```python
from build123d import *

# Parameters (mm, degrees)
BOSS_EXTRUDE1_DEPTH      = 127
BOSS_EXTRUDE1_DEPTH_BACK = 127
SKETCH3_W                = 31.75
SKETCH3_H                = 31.75
SKETCH3_W_2              = 25.4
SKETCH3_H_2              = 25.4
F_10_CLEARANCE_HOLE1_D   = 4.9784
SKETCH7_R                = 14.2875
CUT_EXTRUDE1_DEPTH       = 7.62
CUT_EXTRUDE2_START       = -7.62
SKETCH8_R                = 14.2875
CUT_EXTRUDE2_DEPTH       = 7.62
CUT_EXTRUDE3_DEPTH       = 132.867653824
F_10_CLEARANCE_HOLE2_D   = 4.9784
SKETCH13_R               = 6.35
CUT_EXTRUDE4_DEPTH       = 132.867653824


with BuildPart() as part:
    # Sketch3 → Boss-Extrude1 (new, two sides: drawn at the far end of the back side and taken through both)
    with BuildSketch(Plane.XY.offset(-BOSS_EXTRUDE1_DEPTH_BACK)):
        Rectangle(SKETCH3_W, SKETCH3_H)
        Rectangle(SKETCH3_W_2, SKETCH3_H_2, mode=Mode.SUBTRACT)
    extrude(amount=BOSS_EXTRUDE1_DEPTH + BOSS_EXTRUDE1_DEPTH_BACK)

    # #10 Clearance Hole1 (through all)
    with Locations(Plane(origin=(0, 15.875, 0), x_dir=(1, 0, 0), z_dir=(0, 1, 0))):
        with Locations((-11.1125, -117.475), (11.1125, -117.475), (0, -98.247200001), (-7.111939052, -75.171256705)):
            Hole(F_10_CLEARANCE_HOLE1_D / 2)

    # Sketch7 → Cut-Extrude1 (cut)
    with BuildSketch(Plane(origin=(0, 15.875, 0), x_dir=(1, 0, 0), z_dir=(0, 1, 0))):
        with Locations(Location((0, 17.8816, 0), (0, 0, 270))):
            Circle(SKETCH7_R)
    extrude(amount=-CUT_EXTRUDE1_DEPTH, mode=Mode.SUBTRACT)

    # Sketch8 → Cut-Extrude2 (cut)
    with BuildSketch(Plane.XZ.offset(15.875).offset(CUT_EXTRUDE2_START)):
        with Locations(Location((0, -17.8816, 0), (0, 0, 90))):
            Circle(SKETCH8_R)
    extrude(amount=CUT_EXTRUDE2_DEPTH, mode=Mode.SUBTRACT)

    # Sketch9 → Cut-Extrude3 (cut, through all)
    with BuildSketch(Plane.XZ.offset(15.875)):
        with BuildLine():
            Line((-9.525, 27.51353779), (-9.525, 14.81353779))
            ThreePointArc((-9.525, 14.81353779), (-11.384871939, 10.323409729), (-15.875, 8.46353779))
            Line((-15.875, 8.46353779), (-15.875, 33.86353779))
            ThreePointArc((-15.875, 33.86353779), (-11.384871939, 32.00366585), (-9.525, 27.51353779))
        make_face()
    extrude(amount=-CUT_EXTRUDE3_DEPTH, mode=Mode.SUBTRACT)

    # #10 Clearance Hole2 (through all)
    with Locations(Plane(origin=(15.875, 0, 0), x_dir=(0, 0, -1), z_dir=(1, 0, 0))):
        with Locations((-82.55, 3.175), (114.3, 3.175), (40.132, 3.175)):
            Hole(F_10_CLEARANCE_HOLE2_D / 2)

    # Sketch13 → Cut-Extrude4 (cut, through all)
    with BuildSketch(Plane.XZ.offset(15.875)):
        with Locations((-20.955, 94.525686877)):
            Circle(SKETCH13_R)
    extrude(amount=-CUT_EXTRUDE4_DEPTH, mode=Mode.SUBTRACT)


solid = part.part
```
The listing builds one solid part. Answer for the finished solid, in the listing's coordinates (mm). A direction names the side the tool comes from. Coordinates: 2 decimals unless noted, no trailing zeros. Order: outer loops, then holes, each group sorted by start corner. A loop starts at its lowest first (then second) coordinate and runs counter-clockwise, first axis right, second up. Notation, with made-up numbers: M -2,50.25 L 34,50.25 A13 ccw 34,68.25 Z; hole C 45,82 d6. An arc over 180 degrees is marked long. Answer as a JSON object with one key per item and string values. Group by question number.
1. Determine the mould class of faces 5 (the flat face through (-15.875, 0, 112)), 6 (the cylindrical face through (-8.45, -14.31, 73.07)), 7 (the flat face through (-14, 0, -127)) for opening direction X: released by +X, released by -X, zero draft, split by the parting line, or undercut.
2. Section B-B on x = 0 is taken. Write down the section's boundary in (y, z) (3 decimals), then the cut area to 3 significant figures.
3. A tool of negligible diameter and unlimited length cuts with its end or side. For faces 1 (the flat face through (-12.7, 0, 123)), 2 (the cylindrical face through (0.54, 14.265, 100.677)), 3 (the cylindrical face through (-13.255, -0.222, 33.298)), 4 (the cylindrical face through (-0.628, -13.705, -32.155)), from which of +Z, -Z, +X, -X, +Y, -Y can it reach the whole face along a straight path? Write none if from no direction.
4. Section D-D on z = -78 is taken. Write down the section's boundary in (x, y) (3 decimals), then the cut area to 3 significant figures.
5. Flat-ended cylindrical pins translate along their axes: P1, Ø4, axis at y = 3.175, z = -114.3, coming from the -X side; P2, Ø0.8, axis at x = 13.5, z = -16, coming from the +Y side (3 decimals); P3, Ø2.5, axis at y = -14.5, z = 21, coming from the -X side (3 decimals); P4, Ø0.8, axis at x = 13, z = -20, coming from the -Y side (3 decimals). Find the tip coordinate at first contact, or state that the pin passes through.
6. Straight lines are drawn through the part: line 1 (Y direction, x = -3, z = -98) (3 decimals); line 2 (Z direction, x = 1.5, y = 14). For each, find the intervals that lie inside material, in ascending order.
7. Section A-A on z = -114.3 is taken. Write down the section's boundary in (x, y) (3 decimals), then the cut area to 3 significant figures.
8. Section C-C on y = -1.5 is taken. State how many separate pieces and enclosed holes the cut face has, then the cut area to 3 significant figures.
Values follow:
{
 "1": {"face 5": "released by -X", "face 6": "undercut", "face 7": "zero draft"},
 "2": {"outline": "M -15.875,-127 L -12.7,-127 L -12.7,-32.169 L -15.875,-32.169 Z; M -15.875,-3.594 L -12.7,-3.594 L -12.7,95.758 L -15.875,95.758 Z; M -15.875,100.736 L -12.7,100.736 L -12.7,127 L -15.875,127 Z; M 12.7,-127 L 15.875,-127 L 15.875,-32.169 L 12.7,-32.169 Z; M 12.7,-3.594 L 15.875,-3.594 L 15.875,95.758 L 12.7,95.758 Z; M 12.7,100.736 L 15.875,100.736 L 15.875,127 L 12.7,127 Z", "area": "1,400 mm2"},
 "3": {"face 1": "+Z, -Z", "face 2": "+Y, -Y", "face 3": "-X, +Y, -Y", "face 4": "-Y"},
 "4": {"outline": "M -15.875,-15.875 L 15.875,-15.875 L 15.875,15.875 L -15.875,15.875 Z; hole M -12.7,-12.7 L 12.7,-12.7 L 12.7,12.7 L -12.7,12.7 Z", "area": "363 mm2"},
 "5": {"P1": "through", "P2": "y = 8.255", "P3": "x = -9.525", "P4": "y = -8.255"},
 "6": {"line 1": "-15.875 to -12.7, 12.7 to 15.875", "line 2": "-127 to -32.09, -3.67 to 96.26, 100.23 to 127"},
 "7": {"outline": "M -15.875,-15.875 L 15.875,-15.875 L 15.875,0.686 L 12.7,0.686 L 12.7,-12.7 L -12.7,-12.7 L -12.7,0.686 L -15.875,0.686 Z; M -15.875,5.664 L -12.7,5.664 L -12.7,12.7 L 12.7,12.7 L 12.7,5.664 L 15.875,5.664 L 15.875,15.875 L -15.875,15.875 Z", "area": "331 mm2"},
 "8": {"separate pieces": "3", "enclosed holes": "0", "area": "1,520 mm2"}
}
